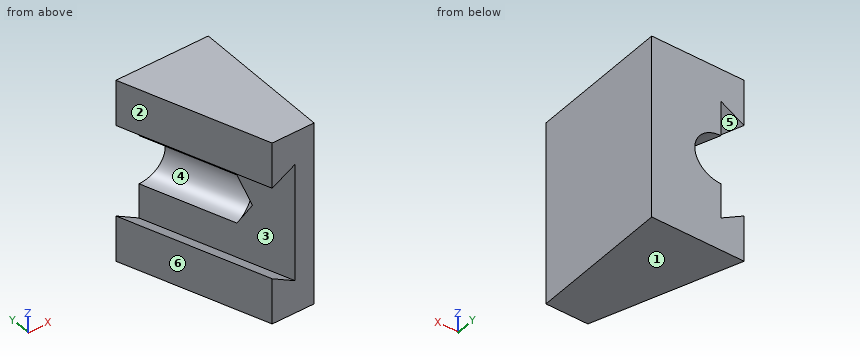
Autodesk Inventor part; units mm, degrees
ref_plane "Work Plane5" through (3.175, 0, -25.4) normal (-0.3420201, 0.9396926, 0) x (0, 0, 1)
ref_plane "YZ Plane" through (0, 0, 0) normal (1, 0, 0) x (0, 1, 0)
ref_plane "XZ Plane" through (0, 0, 0) normal (0, 1, 0) x (-1, 0, 0)
sketch "Sketch1" plane through (0, 0, 0) normal (0, 1, 0) x (-1, 0, 0)
  line L0 (0, 0) -> (-12.7, 0)
  line L1 (-12.7, 0) -> (-12.7, -25.4)
  line L2 (-12.7, -25.4) -> (0, -25.4)
  line L3 (0, -25.4) -> (0, 0)
  line L4 (0, -12.7) -> (-12.7, -12.7) construction
  line L5 (-3.175, -25.4) -> (-3.175, 0)
  line L6 (-3.175, -20.8831) -> (0, -19.05)
  line L7 (-3.175, -4.5169) -> (0, -6.35)
  point P0 (-3.175, -12.7)
  point P1 (0, -6.35)
  dimension "d0" = 12.7
  dimension "d7" = 25.4
  dimension "d34" = 3.175
  dimension "d35" = 60
  dimension "d36" = 12.7
extrude "Extrusion2" add sketch "Sketch1" against normal blind 19.05
sketch "Sketch6" plane through (0, 0, 0) normal (0, 0, 1) x (-1, 0, 0)
  line L0 (0, 0) -> (-12.7, 0)
  line L1 (-12.7, 0) -> (-12.7, 19.05)
  line L2 (-12.7, 19.05) -> (0, 19.05)
  line L3 (0, 0) -> (0, 19.05)
  line L4 (0, 0) -> (-6.9336, 19.05)
  dimension "d41" = 70
sweep "Sweep2" cut profiles "Sketch1" path "Sketch6" path curves L4 contours L3 L6 L5 L7
ref_plane "Work Plane5" through (3.175, 0, -25.4) normal (-0.3420201, 0.9396926, 0) x (0, 0, 1)
ref_plane "Work Plane4" through (0, 0, -25.4) normal (0.9396926, 0.3420201, 0) x (0, 0, 1)
sketch "Sketch7" plane through (3.175, 0, -25.4) normal (-0.3420201, 0.9396926, 0) x (0, 0, 1)
  point P0 (12.7, 0)
hole "Hole3" at (3.175, 0, -12.7) direction (0.3420201, -0.9396926, 0) diameter 6.7564 depth 12.7 tip angle 118
split "Split2" plane through (0, 0, -25.4) removes the side toward (-0.9396926, -0.3420201, 0)
equation "\"d41\" = slopeAngle"
equation "\"slopeAngle\" = 70deg"
equation "\"d44\" = -slopeAngle"
properties material "Steel, Alloy"
The listing builds one solid part. Answer for the finished solid, in the listing's coordinates (mm). Face numbers are marked on the shaded views. A direction names the side the tool comes from. Round coordinates to 2 decimals unless told otherwise and drop trailing zeros. Loops run counter-clockwise (first coordinate to the right, second up) from the corner with the lowest first, then second, coordinate; pieces in that order, holes last.
Q1. Section C-C, the plane z = -22.5 is taken. Determine the outline of the cut face in (x, y).
Q2. Given pin 1 Ø6 at (x, y) = (7.5, -5) entering from +Z; pin 2 Ø3 at (y, z) = (-17, -17) entering from -X, each flat-ended and moving along its own axis, determine where each tip first touches the part or whether it passes through.
Q3. Find the intervals of material crossed by line 1 (Z direction, x = 4.5, y = -9.5); line 2 (Z direction, x = 7.5, y = -3); line 3 (X direction, y = -8.25, z = -4.75), in increasing order.
Q4. Which of the six approach directions +Z, -Z, +X, -X, +Y, -Y give full straight-line access (tool end or side, diameter ignored) to the marked faces 4, 5 and 6?
Q5. Section A-A, the plane x = 2 is taken. Determine the outline of the cut face in (y, z), then the cut area to 3 significant figures.
Q6. For a pull along Z with two mould halves and no side action, classify the marked faces 1, 2 and 3 as released by +Z, released by -Z, zero draft, split by the parting line, or undercut.
Q7. Section B-B, the plane z = -9 is taken. Determine the outline of the cut face in (x, y) (3 decimals).
Completed:
1. outline: (0, 0) - (6.93, -19.05) - (12.7, -19.05) - (12.7, 0) - close
2. pin 1: stops at z = 0
2. pin 2: stops at x = 8.82
3. line 1: z = -25.4 to -19.65, -5.75 to 0
3. line 2: z = -25.4 to -14.18, -11.22 to 0
3. line 3: x = 3 to 5.77, 6.18 to 12.7
4. face 4: -X
4. face 5: none
4. face 6: +Z, -Z, -X, -Y
5. outline: (-5.49, -25.4) - (0, -25.4) - (0, -20.2) - (-5.49, -19.05) - close; (-5.49, -6.35) - (0, -5.2) - (0, 0) - (-5.49, 0) - close
5. area: 63.4 mm2
6. face 1: released by -Z
6. face 2: zero draft
6. face 3: undercut
7. outline: (3.175, 0) - (10.109, -19.05) - (12.7, -19.05) - (12.7, 0) - close
